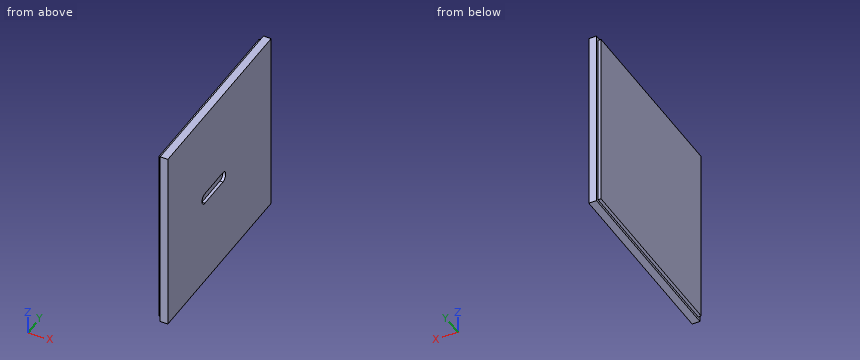
from build123d import *

# Parameters (mm, degrees)
F0_W     = 326
F0_H     = 314
F1_DEPTH = 18
F3_DEPTH = 5
F4_W     = 326
F4_H     = 314
F4_W_2   = 316
F4_H_2   = 304
F5_DEPTH = 5


with BuildPart() as f1:
    # F0 (on Right) → F1 (new body)
    with BuildSketch(Plane.YZ):
        Rectangle(F0_W, F0_H)
    extrude(amount=-F1_DEPTH)

    # F2 (on face) → F3 (cut)
    with BuildSketch(Plane.YZ):
        with BuildLine():
            ThreePointArc((10.5, -9), (19.5, 0), (10.5, 9))
            Line((10.5, 9), (-46.5, 9))
            ThreePointArc((-46.5, 9), (-55.5, 0), (-46.5, -9))
            Line((-46.5, -9), (10.5, -9))
        make_face()
    extrude(amount=-F3_DEPTH, mode=Mode.SUBTRACT)

    # F4 (on face) → F5 (cut)
    with BuildSketch(Plane(origin=(-18, 0, 0), x_dir=(0, -1, 0), z_dir=(-1, 0, 0))):
        Rectangle(F4_W, F4_H)
        Rectangle(F4_W_2, F4_H_2, mode=Mode.SUBTRACT)
    extrude(amount=-F5_DEPTH, mode=Mode.SUBTRACT)


solid = f1.part
Read the model definition and answer for the solid it produces. Units are mm, in the model's axes. Give positions to 0.01 mm unless a question says otherwise; leave off trailing zeros. Write each loop counter-clockwise with the first axis right and the second up, starting at its lowest first coordinate (ties: lowest second). Pieces come first, ordered by that corner, then holes. Notation, with made-up numbers: (84, 59) -> (103, 59) arc R22 cw to (103, 72) -> close; hole circle Ø10 at (69.25, 12). An arc over 180 degrees is marked (long way). Answer as a JSON object with one key per item and string values. Group by question number.
1) Consider L1, parallel to Z at x = -1, y = -1; L2, parallel to Y at x = -16, z = -30.5; L3, parallel to Z at x = -15.5, y = -131. Determine where each line is inside the solid, lowest interval first. Write a range as from..to.
2) Find section A-A (z = 0). Write down the section's boundary in (x, y).
3) Each of these flat-tipped pins is pushed along its axis until it touches: P1, Ø10, axis at y = 6.5, z = -10, coming from the +X side; P2, Ø1.5, axis at x = -16.5, y = -53, coming from the -Z side; P3, Ø1.5, axis at x = -16.5, z = 12.5, coming from the -Y side; P4, Ø1.5, axis at x = -15, z = 67, coming from the +Y side. Where does it stop, or does it pass through?
Values follow:
{
 "1": {"L1": "z = -157..-9, 9..157", "L2": "y = -158..158", "L3": "z = -152..152"},
 "2": {"outline": "(-18, -158) -> (-13, -158) -> (-13, -163) -> (0, -163) -> (0, -55.5) -> (-5, -55.5) -> (-5, 19.5) -> (0, 19.5) -> (0, 163) -> (-13, 163) -> (-13, 158) -> (-18, 158) -> close"},
 "3": {"P1": "stops at x = 0", "P2": "stops at z = -152", "P3": "stops at y = -158", "P4": "stops at y = 158"}
}
